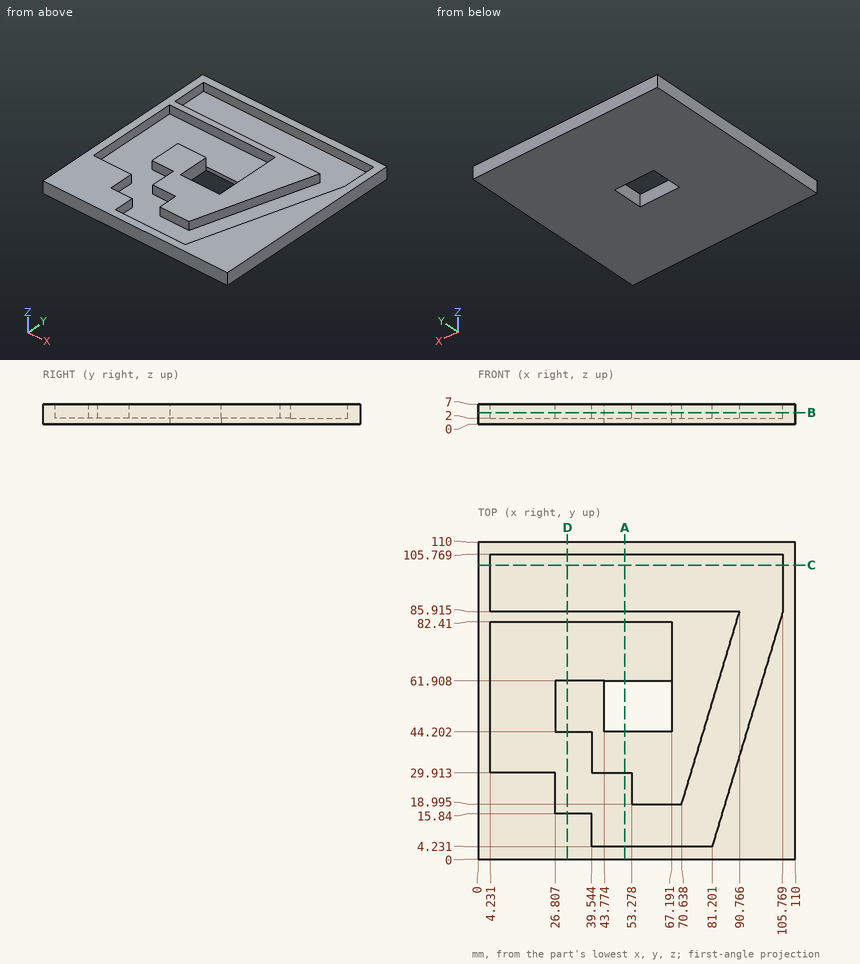
Geometry check sheet. Reference: drawing and pictorial views, mm from the part's lowest x, y, z. Coordinates: 2 decimals unless noted, no trailing zeros. Order: outer loops, then holes, each group sorted by start corner. A loop starts at its lowest first (then second) coordinate and runs counter-clockwise, first axis right, second up.
Item 1: Section check D-D (x = 31). Enter the section's corners in (y, z) (1 decimal).
Item 2: Section check B-B (z = 4). Enter the section's corners in (x, y) (1 decimal), plus the area to 3 significant figures.
Item 3: Section check A-A (x = 51). Enter the section's corners in (y, z) (1 decimal).
Item 4: Depth check by flat-ended pin: pin 1 (2.5 mm diameter, centred on x = 33.5, z = 3.5, fed in from -Y). Enter the tip coordinate at first touch or a pass-through.
Item 5: Scan lines: line 1 along Y through (x, z) = (57, 6) (1 decimal); line 2 along Y through (x, z) = (49.5, 4) (1 decimal); line 3 along Y through (x, z) = (18, 5.25) (1 decimal). Record each from-to range of solid material in increasing order.
Item 6: Section check C-C (y = 102). Enter the section's corners in (x, z).
Check sheet entries:
1. outline: (0, 0) - (110, 0) - (110, 7) - (105.8, 7) - (105.8, 2) - (85.9, 2) - (85.9, 7) - (82.4, 7) - (82.4, 2) - (61.9, 2) - (61.9, 7) - (44.2, 7) - (44.2, 2) - (15.8, 2) - (15.8, 7) - (0, 7) - close
2. outline: (0, 0) - (110, 0) - (110, 110) - (0, 110) - close; hole (4.2, 29.9) - (26.8, 29.9) - (26.8, 15.8) - (39.5, 15.8) - (39.5, 4.2) - (81.2, 4.2) - (105.8, 85.9) - (105.8, 105.8) - (4.2, 105.8) - (4.2, 85.9) - (90.8, 85.9) - (70.6, 19) - (53.3, 19) - (53.3, 29.9) - (39.5, 29.9) - (39.5, 44.2) - (26.8, 44.2) - (26.8, 61.9) - (43.8, 61.9) - (43.8, 44.2) - (67.2, 44.2) - (67.2, 82.4) - (4.2, 82.4) - close
2. area: 5,490 mm2
3. outline: (0, 0) - (44.2, 0) - (44.2, 7) - (29.9, 7) - (29.9, 2) - (4.2, 2) - (4.2, 7) - (0, 7) - close; (61.9, 0) - (110, 0) - (110, 7) - (105.8, 7) - (105.8, 2) - (85.9, 2) - (85.9, 7) - (82.4, 7) - (82.4, 2) - (61.9, 2) - close
4. pin 1: stops at y = 0
5. line 1: y = 0 to 4.2, 19 to 44.2, 82.4 to 85.9, 105.8 to 110
5. line 2: y = 0 to 4.2, 29.9 to 44.2, 82.4 to 85.9, 105.8 to 110
5. line 3: y = 0 to 29.9, 82.4 to 85.9, 105.8 to 110
6. outline: (0, 0) - (110, 0) - (110, 7) - (105.77, 7) - (105.77, 2) - (4.23, 2) - (4.23, 7) - (0, 7) - close
